Read the model definition and answer for the solid it produces. Units are mm, in the model's axes. Face numbers are marked on the shaded views. A direction names the side the tool comes from. Coordinates: 2 decimals unless noted, no trailing zeros. Loops run counter-clockwise (first coordinate to the right, second up) from the corner with the lowest first, then second, coordinate; pieces in that order, holes last.
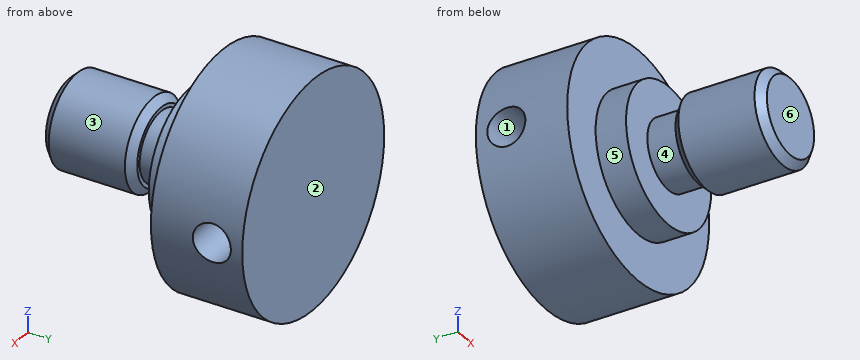
Autodesk Inventor part; units mm, degrees
ref_plane "YZ Plane" through (0, 0, 0) normal (1, 0, 0) x (0, 1, 0)
ref_plane "XZ Plane" through (0, 0, 0) normal (0, 1, 0) x (-1, 0, 0)
ref_plane "XY Plane" through (0, 0, 0) normal (0, 0, 1) x (1, 0, 0)
sketch "Sketch3" plane through (0, 0, 0) normal (0, 0, 1) x (1, 0, 0)
  line L0 (0, 3) -> (7.5, 3)
  line L1 (7.5, 3) -> (7.5, -3)
  line L2 (7.5, -3) -> (4.5, -3)
  line L3 (4.5, -3) -> (4.5, -5)
  line L4 (4.5, -5) -> (3, -5)
  line L5 (0, -16.2) -> (0, 6.2)
  line L6 (3, -5) -> (3, -13)
  line L7 (3, -13) -> (0, -13)
  point P0 (0, 0)
  point P1 (7.5, 0)
  dimension "d6" = 6
  dimension "d7" = 15
  dimension "d8" = 9
  dimension "d9" = 2
  dimension "d11" = 6
  dimension "d12" = 8
revolve "Revolution1" add sketch "Sketch3" angle 360 about axis through (0, -10, 0) along (0, 1, 0)
sketch "Sketch4" plane through (0, 0, 0) normal (1, 0, 0) x (0, 1, 0)
  circle A0 centre (1, 0) radius 1.25
  line L0 (3, 7.5) -> (3, -7.5)
  point P0 (0, 0)
  dimension "d13" = 2.5
  dimension "d14" = 2
extrude "Extrusion3" cut sketch "Sketch4" along normal through all both and the other way through all
sketch "Sketch5" plane through (0, 0, 0) normal (1, 0, 0) x (0, 1, 0)
  line L0 (-7, 2.25) -> (-5, 2.25)
  line L1 (-5, 2.25) -> (-5, 3)
  line L2 (-5, 3) -> (-7, 3)
  line L3 (-7, 3) -> (-7, 2.25)
  line L4 (-5, 3) -> (-13, 3)
  line L5 (-5, 4.5) -> (-5, -4.5)
  line L6 (-16.2, 0) -> (6.2, 0)
  point P0 (0, 0)
  dimension "d17" = 2
  dimension "d18" = 4.5
revolve "Revolution2" cut sketch "Sketch5" angle 360 about axis through (0, -10, 0) along (0, 1, 0)
thread "Thread1"
chamfer "Chamfer1" distance 0.5 angle 45 2 edges at (-3, -13, 0) (-3, -7, 0)
properties part number "Thumb Screw" material "Steel, Mild"
Q1. A cutting plane is placed at D-D (z = -4.25). Give the vertices of the cut face in (x, y), then the cut area to 3 significant figures.
Findings below:
outline: (-6.18, -3) - (-1.48, -3) - (-1.48, -5) - (1.48, -5) - (1.48, -3) - (6.18, -3) - (6.18, 3) - (-6.18, 3) - close
area: 80.1 mm2
Q2. Which of the six approach directions +Z, -Z, +X, -X, +Y, -Y give full straight-line access (tool end or side, diameter ignored) to the marked faces 4, 5 and 6?
Findings below:
face 4: none
face 5: -Y
face 6: +Z, -Z, +X, -X, -Y
Q3. A cutting plane is placed at A-A (z = 0). Give the vertices of the cut face in (x, y), then the cut area to 3 significant figures.
Findings below:
outline: (-7.5, -3) - (-4.5, -3) - (-4.5, -5) - (-2.25, -5) - (-2.25, -7) - (-2.5, -7) - (-3, -7.5) - (-3, -12.5) - (-2.5, -13) - (2.5, -13) - (3, -12.5) - (3, -7.5) - (2.5, -7) - (2.25, -7) - (2.25, -5) - (4.5, -5) - (4.5, -3) - (7.5, -3) - (7.5, -0.25) - (-7.5, -0.25) - close; (-7.5, 2.25) - (7.5, 2.25) - (7.5, 3) - (-7.5, 3) - close
area: 115 mm2
Q4. Flat-ended cylindrical pins translate along their axes: pin 1 Ø5 at (x, z) = (6, -2) entering from -Y; pin 2 Ø2 at (x, z) = (-2.5, 3) entering from -Y; pin 3 Ø3 at (x, y) = (-3.5, 0.5) entering from -Z; pin 4 Ø2 at (y, z) = (1, 0) entering from +X. Find the tip coordinate at first contact, or state that the pin passes through.
Findings below:
pin 1: stops at y = -5
pin 2: stops at y = -12.59
pin 3: stops at z = -7.23
pin 4: passes through
Q5. Straight lines are drawn through the part: probe 1 along Y at (x, z) = (-2.75, 0); probe 2 along Y at (x, z) = (-3, 4); probe 3 along Y at (x, z) = (-0.75, 0). For each, find the intervals that lie inside material, in ascending order.
Findings below:
probe 1: y = -12.75 to -7.25, -5 to -0.25, 2.25 to 3
probe 2: y = -3 to 3
probe 3: y = -13 to -0.25, 2.25 to 3
Q6. Determine the mould class of the marked faces 1, 2 and 3 for opening direction Z: +Z half, -Z half, draft (parallel to the pull), parting line (faces both ways), or undercut.
Findings below:
face 1: undercut
face 2: draft
face 3: parting line
Q7. A cutting plane is placed at C-C (y = -6.75). Give the vertices of the cut face in (x, z).
Findings below:
outline: circle Ø4.5 at (0, 0)
Q8. A cutting plane is placed at B-B (x = 0). Give the vertices of the cut face in (y, z).
Findings below:
outline: (-13, -2.5) - (-12.5, -3) - (-7.5, -3) - (-7, -2.5) - (-7, -2.25) - (-5, -2.25) - (-5, -4.5) - (-3, -4.5) - (-3, -7.5) - (3, -7.5) - (3, 7.5) - (-3, 7.5) - (-3, 4.5) - (-5, 4.5) - (-5, 2.25) - (-7, 2.25) - (-7, 2.5) - (-7.5, 3) - (-12.5, 3) - (-13, 2.5) - close; hole circle Ø2.5 at (1, 0)
